Input: part model. Units: mm. Frame: model coordinates. A direction names the side the tool comes from. Give positions to 0.01 mm unless a question says otherwise; leave off trailing zeros. Loops run counter-clockwise (first coordinate to the right, second up) from the corner with the lowest first, then second, coordinate; pieces in that order, holes last. Notation, with made-up numbers: M 12.5,71 L 54.5,71 A18 ccw 54.5,94 Z; hole C 50,-36 d10. An arc over 180 degrees is marked long. One line per item, written item: value. Start each with the question number.
(1) Pull-direction query (Y, two-part tool) for faces 1 (the flat face through (-15, -6.35, -14)), 2 (the flat face through (-2, -3, -14)), 3 (the flat face through (11, -6, -21.7)); classes: released by +Y, released by -Y, zero draft, split by the parting line, or undercut.
(2) Section C-C on z = -14.5. Output: boundary loops of the cut face in (x, y) (3 decimals), plus the area to 3 significant figures.
(3) Section B-B on x = -15.5. Output: boundary loops of the cut face in (y, z), plus the area to 3 significant figures.
(4) Pin query (flat end, axial travel): P1, Ø7.5, axis at x = 7.625, y = -6.35, coming from the +Z side; P2, Ø6, axis at x = -14, z = -7.5, coming from the +Y side; P3, Ø5, axis at x = -5.625, z = -20.7, coming from the -Y side. Return the tip coordinate at first contact, or that it passes through.
(5) Ray query, line 1 along X through (y, z) = (-8.2, -7) (3 decimals); line 2 along X through (y, z) = (-7.8, -20.7) (3 decimals); line 3 along Z through (x, y) = (-8, -11). Return the intervals inside material, ascending. Write a range as from..to.
(6) Access query for faces 4 (the flat face through (5, 0, -19)), 5 (the cylindrical face through (10.358, -6.957, -17.137)), 6 (the flat face through (8, -3, -12.7)), 7 (the flat face through (-9.25, -7, -13)), 8 (the flat face through (-12.9, -11.22, -8.41)). Directions: +Z, -Z, +X, -X, +Y, -Y. A direction counts if a zero-diameter tool reaches every point of the face in a straight line with its end or side. Return the directions, or none.
(7) Section A-A on y = -12. State how many separate pieces and enclosed holes the cut face has, plus the area to 3 significant figures.
(8) Section D-D on y = -8.25. Output: boundary loops of the cut face in (x, z) (3 decimals).
Autodesk Inventor part; units mm, degrees
ref_plane "Arbeitsebene1" through (0, 0, -12.7) normal (0, 0, -1) x (-1, 0, 0)
ref_plane "YZ Plane" through (0, 0, 0) normal (1, 0, 0) x (0, 1, 0)
ref_plane "XZ Plane" through (0, 0, 0) normal (0, 1, 0) x (-1, 0, 0)
ref_plane "Arbeitsebene1" through (0, 0, -12.7) normal (0, 0, -1) x (-1, 0, 0)
sketch "Skizze2" plane through (0, 0, -12.7) normal (0, 0, -1) x (-1, 0, 0)
  line L0 (-55.25, 0) -> (-55.25, -12.7)
  line L1 (0, -12.7) -> (-55.25, -12.7)
  line L2 (0, 0) -> (0, -12.7)
  line L3 (0, 0) -> (-55.25, 0)
  circle A0 centre (-47.625, -6.35) radius 2.75
  circle A1 centre (-7.625, -6.35) radius 2.75
  line L4 (0, 1.15) -> (-15, 1.15)
  line L5 (-15, 1.15) -> (-15, -13.85)
  line L6 (-15, -13.85) -> (0, -13.85)
  line L7 (0, -13.85) -> (0, 1.15)
  point P0 (-15, -6.35)
  dimension "d1" = 15
  dimension "d2" = 0
  dimension "d3" = 15
extrude "Extrusion1" add sketch "Skizze2" along normal blind 15 contours L5 L4 L7 L3 | L3 L2 L1 L5 | L1 L7 L6 L5 | A1
sketch "Skizze3" plane through (0, -13.85, -12.7) normal (-1, 0, 0) x (0, 0, 1)
  line L0 (12.7, 1.15) -> (12.7, 13.85)
  line L1 (-15, 0) -> (-15, 15)
  line L2 (-15, 15) -> (12.7, 15)
  line L3 (12.7, 15) -> (12.7, 0)
  line L4 (12.7, 0) -> (-15, 0)
  line L5 (-15, 0) -> (-15, 15)
  line L6 (0, 0) -> (-15, 0)
extrude "Extrusion2" add sketch "Skizze3" along normal blind 2
sketch "Skizze4" plane through (-2, -13.85, -12.7) normal (-1, 0, 0) x (0, 0, 1)
  line L0 (0, 0) -> (12.7, 0)
  line L1 (-15, 15) -> (-15, 0)
  line L2 (12.7, 0) -> (-15, 0)
  line L3 (-15, 0) -> (-15, 7.5)
  line L4 (-15, 7.5) -> (12.7, 7.5)
  line L5 (12.7, 7.5) -> (12.7, 0)
  line L6 (12.7, 0) -> (12.7, 15)
  point P0 (12.7, 13.85)
  point P1 (12.7, 7.5)
  point P2 (-1.15, 7.5)
extrude "Extrusion3" add sketch "Skizze4" along normal blind 17
sketch "Skizze5" plane through (-2, -6.35, 0) normal (0, 1, 0) x (1, 0, 0)
  line L0 (0, 27.7) -> (-17, 27.7)
  line L1 (0, 0) -> (0, 27.7)
  line L2 (0, 0) -> (-17, 0)
  line L3 (-17, 0) -> (-17, 27.7)
  line L4 (-7.25, 0) -> (-9.75, 0)
  line L5 (-9.75, 0) -> (-9.75, 25.75)
  line L6 (-9.75, 25.75) -> (-7.25, 25.75)
  line L7 (-7.25, 25.75) -> (-7.25, 0)
  point P0 (2, 0)
  point P1 (-8.5, 0)
  point P2 (-8.5, 0)
  dimension "d10" = 2.5
  dimension "d17" = 25.75
extrude "Extrusion4" cut sketch "Skizze5" against normal blind 1.25 contours L2 L5 L6 L7
sketch "Skizze6" plane through (-2, -6.35, 0) normal (0, 1, 0) x (1, 0, 0)
  line L0 (-9.75, 25.75) -> (-7.25, 25.75)
  line L1 (-7.25, 25.75) -> (-7.25, 0)
  line L2 (-9.75, 0) -> (-9.75, 25.75)
  line L3 (0, 27.7) -> (-17, 27.7)
  line L4 (-9.75, 25.75) -> (-7.25, 25.75)
  line L5 (-7.8, 25.75) -> (-9.2, 25.75)
  line L6 (-9.2, 25.75) -> (-9.2, 27.7)
  line L7 (-9.2, 27.7) -> (-7.8, 27.7)
  line L8 (-7.8, 27.7) -> (-7.8, 25.75)
  point P0 (2, 0)
  point P1 (-8.5, 25.75)
  point P2 (-8.5, 25.75)
  point P3 (-7.8, 27.7)
  dimension "d14" = 1.4
extrude "Extrusion5" cut sketch "Skizze6" against normal blind 0.7
sketch "Skizze7" plane through (-2, -6.35, 0) normal (0, 1, 0) x (1, 0, 0)
  circle A0 centre (-3.625, 7) radius 2
  circle A1 centre (-13.375, 7) radius 2
  circle A2 centre (-13.375, 20.7) radius 2
  circle A3 centre (-3.625, 20.7) radius 2
  line L0 (0, 0) -> (-7.25, 0)
  line L1 (-9.75, 0) -> (-17, 0)
  line L2 (-9.2, 27.7) -> (-17, 27.7)
  point P0 (2, 0)
  point P1 (-3.625, 0)
  point P2 (-13.375, 0)
  dimension "d18" = 4
  dimension "d19" = 4
  dimension "d20" = 4
  dimension "d21" = 4
  dimension "d22" = 7
  dimension "d23" = 7
extrude "Extrusion6" cut sketch "Skizze7" against normal blind 10
sketch "Skizze9" plane through (0, 0, -27.7) normal (0, 0, -1) x (-1, 0, 0)
  circle A0 centre (-7.625, -6.35) radius 2.75
  point P0 (0, 0)
hole "Bohrung1" at (7.625, -6.35, -27.7) direction (0, 0, 1) diameter 5.6 depth 15 counterbore diameter 9 counterbore depth 6
sketch "Skizze10" plane through (0, 1.15, -12.7) normal (0, 1, 0) x (1, 0, 0)
  line L0 (19, -16) -> (-4, -16)
  line L1 (-4, -16) -> (-4, 20)
  line L2 (-4, 20) -> (19, 20)
  line L3 (19, 20) -> (19, -16)
  point P0 (0, -12.7)
extrude "Extrusion8" cut sketch "Skizze10" against normal blind 1.15
sketch "Skizze11" plane through (15, -13.85, -27.7) normal (0, -1, 0) x (1, 0, 0)
  line L0 (6, 49) -> (-39, 49)
  line L1 (-39, 49) -> (-39, -17)
  line L2 (-39, -17) -> (6, -17)
  line L3 (6, -17) -> (6, 49)
  point P0 (-15, 27.7)
extrude "Extrusion9" cut sketch "Skizze11" against normal blind 1.15
fillet "Rundung2" radius 2 5 edges at (-19, -9.525, -27.7) (-19, -9.525, 0) (15, -6.35, -27.7) (15, 0, -20.2) (6.5, 0, -27.7)
sketch "Skizze12" plane through (15, -12.7, -27.7) normal (0, -1, 0) x (1, 0, 0)
  circle A0 centre (-30.375, 20.7) radius 2
  circle A1 centre (-20.625, 20.7) radius 2
  circle A2 centre (-20.625, 7) radius 2
  circle A3 centre (-30.375, 7) radius 2
  line L0 (-27.0841, 20.7) -> (-28.7296, 17.85)
  line L1 (-28.7296, 17.85) -> (-32.0204, 17.85)
  line L2 (-32.0204, 17.85) -> (-33.6659, 20.7)
  line L3 (-33.6659, 20.7) -> (-32.0204, 23.55)
  line L4 (-32.0204, 23.55) -> (-28.7296, 23.55)
  line L5 (-28.7296, 23.55) -> (-27.0841, 20.7)
  line L6 (-17.3341, 20.7) -> (-18.9796, 17.85)
  line L7 (-18.9796, 17.85) -> (-22.2704, 17.85)
  line L8 (-22.2704, 17.85) -> (-23.9159, 20.7)
  line L9 (-23.9159, 20.7) -> (-22.2704, 23.55)
  line L10 (-22.2704, 23.55) -> (-18.9796, 23.55)
  line L11 (-18.9796, 23.55) -> (-17.3341, 20.7)
  line L12 (-17.3341, 7) -> (-18.9796, 4.15)
  line L13 (-18.9796, 4.15) -> (-22.2704, 4.15)
  line L14 (-22.2704, 4.15) -> (-23.9159, 7)
  line L15 (-23.9159, 7) -> (-22.2704, 9.85)
  line L16 (-22.2704, 9.85) -> (-18.9796, 9.85)
  line L17 (-18.9796, 9.85) -> (-17.3341, 7)
  line L18 (-28.7296, 4.15) -> (-32.0204, 4.15)
  line L19 (-32.0204, 4.15) -> (-33.6659, 7)
  line L20 (-33.6659, 7) -> (-32.0204, 9.85)
  line L21 (-32.0204, 9.85) -> (-28.7296, 9.85)
  line L22 (-28.7296, 9.85) -> (-27.0841, 7)
  line L23 (-27.0841, 7) -> (-28.7296, 4.15)
  line L24 (-2, 0) -> (-32, 0)
  point P0 (-15, 27.7)
  point P1 (-30.375, 17.85)
  point P2 (-20.625, 17.85)
  dimension "d43" = 5.7
extrude "Extrusion10" cut sketch "Skizze12" against normal blind 3 contours A1 | A2 | A3 | L0 L1 L2 L3 L4 L5 | L6 L7 L8 L9 L10 L11 | L12 L13 L14 L15 L16 L17 | L18 L19 L20 L21 L22 L23
equation "\"d19\" = d18"
equation "\"d20\" = d19"
equation "\"d21\" = d19"
equation "\"d23\" = d22"
properties part number "NadelhalterSchraub"
Output values:
1. face 1: released by +Y
1. face 2: zero draft
1. face 3: undercut
2. outline: M -19,-12.7 L 15,-12.7 L 15,-2 A2 ccw 13,0 L -2,0 L -2,-6.35 L -9.25,-6.35 L -9.25,-7.6 L -11.75,-7.6 L -11.75,-6.35 L -19,-6.35 Z; hole C 7.625,-6.35 d5.6
2. area: 295 mm²
3. outline: M -12.7,-27.7 L -6.35,-27.7 L -6.35,-22.7 L -9.7,-22.7 L -9.7,-23.55 L -12.7,-23.55 Z; M -12.7,-17.85 L -9.7,-17.85 L -9.7,-18.7 L -6.35,-18.7 L -6.35,-9 L -9.7,-9 L -9.7,-9.85 L -12.7,-9.85 Z; M -12.7,-4.15 L -9.7,-4.15 L -9.7,-5 L -6.35,-5 L -6.35,0 L -12.7,0 Z
3. area: 115 mm²
4. P1: stops at z = -12.7
4. P2: stops at y = -6.35
4. P3: stops at y = -9.7
5. line 1: x = -19..-17.375, -13.375..-7.625, -3.625..0
5. line 2: x = -19..-17.375, -13.375..-7.625, -3.625..5.23, 10.02..15
5. line 3: z = -27.7..-22.29, -19.11..-8.59, -5.41..0
6. face 4: +Z, -Z, +X, -X, +Y
6. face 5: +Z, -Z
6. face 6: +Z, +X, +Y, -Y
6. face 7: +Z, +Y
6. face 8: -Y
7. separate pieces: 1
7. enclosed holes: 4
7. area: 636 mm²
8. outline: M -19,-25.7 A2 ccw -17,-27.7 L 3.546,-27.7 L 3.546,-21.7 L 5.568,-21.7 L 5.568,-12.7 L 0,-12.7 L 0,0 L -17,0 A2 ccw -19,-2 Z; M 9.682,-21.7 L 11.704,-21.7 L 11.704,-27.7 L 13,-27.7 A2 ccw 15,-25.7 L 15,-12.7 L 9.682,-12.7 Z; hole C -15.375,-20.7 d4; hole C -15.375,-7 d4; hole C -5.625,-20.7 d4; hole C -5.625,-7 d4
